```python
from build123d import *
from OCP.BRepAlgoAPI import BRepAlgoAPI_Cut
from OCP.TopTools import TopTools_ListOfShape

# Parameters (mm, degrees)
EXTRUDE_1_DEPTH        = 5
EXTRUDE_1_DEPTH_BACK   = 280.836309
SKETCH_1_R             = 12.5
HOLE_WIZARD_M101_D     = 8.5
HOLE_WIZARD_M101_DEPTH = 27.5
HOLE_WIZARD_M101_TIP   = 2.553657631
SKETCH_6_W             = 7
SKETCH_6_H             = 7
CUT_EXTRUDE_1_DEPTH    = 35
SKETCH_7_W             = 1.5
SKETCH_7_H             = 2.75
CUT_EXTRUDE_START      = -285.836309
SKETCH_6_2_W           = 7
SKETCH_6_2_H           = 7
CUT_EXTRUDE_2_DEPTH    = 31.8
HOLE_WIZARD_M102_D     = 8.5
HOLE_WIZARD_M102_DEPTH = 27.5
HOLE_WIZARD_M102_TIP   = 2.553657631


with BuildPart() as part:
    # Эскиз1 → Бобышка-Вытянуть1 (new, two sides: drawn at the far end of the back side and taken through both)
    with BuildSketch(Plane.XY.offset(-EXTRUDE_1_DEPTH_BACK)):
        Circle(SKETCH_1_R)
    extrude(amount=EXTRUDE_1_DEPTH + EXTRUDE_1_DEPTH_BACK)

    # Отверстие обработанное метчиком M101
    with Locations(Plane(origin=(0, 0, -280.836309448), x_dir=(-1, 0, 0), z_dir=(0, 0, -1))):
        with Locations((0, 0)):
            Hole(HOLE_WIZARD_M101_D / 2, depth=HOLE_WIZARD_M101_DEPTH)
            with Locations((0, 0, -(HOLE_WIZARD_M101_DEPTH + HOLE_WIZARD_M101_TIP / 2))):  # 118° drill point
                Cone(0, HOLE_WIZARD_M101_D / 2, HOLE_WIZARD_M101_TIP, mode=Mode.SUBTRACT)

    # Эскиз6 → Вырез-Вытянуть1 (cut)
    with BuildSketch(Plane(origin=(0, 0, -280.836309448), x_dir=(-1, 0, 0), z_dir=(0, 0, -1))):
        with Locations((0, 12.5)):
            Rectangle(SKETCH_6_W, SKETCH_6_H)
    extrude(amount=-CUT_EXTRUDE_1_DEPTH, mode=Mode.SUBTRACT)

    # Эскиз7 → Вырез-Повернуть1 (revolve, cut)
    with BuildSketch(Plane(origin=(0, 0, 0), x_dir=(0, 0, -1), z_dir=(1, 0, 0)), mode=Mode.PRIVATE) as cut_revolve_1_sk:
        with Locations((62.65, 13.125)):
            Rectangle(SKETCH_7_W, SKETCH_7_H)
        with Locations((27.55, 13.125)):
            Rectangle(SKETCH_7_W, SKETCH_7_H)
        with Locations((168.386309448, 13.125)):
            Rectangle(SKETCH_7_W, SKETCH_7_H)
    revolve(cut_revolve_1_sk.sketch.rotate(Axis((0, 0, 1000), (0, 0, -1)), 90), axis=Axis((0, 0, 1000), (0, 0, -1)), mode=Mode.SUBTRACT)


with BuildPart() as cut_extrude_2_tool:
    # Эскиз6<2> → Вырез-Вытянуть2 (new body)
    with BuildSketch(Plane(origin=(0, 0, -280.836309448), x_dir=(-1, 0, 0), z_dir=(0, 0, -1)).offset(CUT_EXTRUDE_START)):
        with Locations((0, 12.5)):
            Rectangle(SKETCH_6_2_W, SKETCH_6_2_H)
    extrude(amount=CUT_EXTRUDE_2_DEPTH)


with BuildPart() as part_1:
    add(part.part)

    # Вырез-Вытянуть2: cut by cut_extrude_2_tool, with a tolerance
    cut_extrude_2_stock = TopTools_ListOfShape()
    cut_extrude_2_stock.Append(part_1.part.wrapped)
    cut_extrude_2_tools = TopTools_ListOfShape()
    cut_extrude_2_tools.Append(cut_extrude_2_tool.part.wrapped)
    cut_extrude_2_cut = BRepAlgoAPI_Cut()
    cut_extrude_2_cut.SetArguments(cut_extrude_2_stock)
    cut_extrude_2_cut.SetTools(cut_extrude_2_tools)
    cut_extrude_2_cut.SetFuzzyValue(0.00001)
    cut_extrude_2_cut.Build()
    add(Compound.cast(cut_extrude_2_cut.Shape()).solids(), mode=Mode.REPLACE)

    # Отверстие обработанное метчиком M102
    with Locations(Plane.XY.offset(5)):
        with Locations((0, 0)):
            Hole(HOLE_WIZARD_M102_D / 2, depth=HOLE_WIZARD_M102_DEPTH)
            with Locations((0, 0, -(HOLE_WIZARD_M102_DEPTH + HOLE_WIZARD_M102_TIP / 2))):  # 118° drill point
                Cone(0, HOLE_WIZARD_M102_D / 2, HOLE_WIZARD_M102_TIP, mode=Mode.SUBTRACT)


solid = part_1.part
```
Source: CAD feature listing. Evaluate the final solid. Frame: model axes, mm. A direction names the side the tool comes from. Round coordinates to 2 decimals unless told otherwise and drop trailing zeros. Loops run counter-clockwise (first coordinate to the right, second up) from the corner with the lowest first, then second, coordinate; pieces in that order, holes last.
(1) Contact query for flat-ended pins moving along their axis: pin 1 Ø5.5 at (x, z) = (-1.5, -268.5) entering from +Y; pin 2 Ø10 at (x, z) = (8.5, -148) entering from -Y; pin 3 Ø4 at (y, z) = (6, -112.5) entering from -X. Output: stop coordinate, or through.
From the geometry:
pin 1: stops at y = 12
pin 2: stops at y = -12
pin 3: stops at x = -11.84
(2) Section query A-A (z = -259). Output: boundary loops of the cut face in (x, y), and give its area (3 significant figures).
From the geometry:
outline: (-3.5, 9) - (-3.5, 12) arc R12.5 ccw (long way) to (3.5, 12) - (3.5, 9) - close; hole circle Ø8.5 at (0, 0)
area: 411 mm2
(3) Pull-direction query (Z, two-part tool) for faces 1 (the cylindrical face through (-0.5, -12.49, -11.12)), 2 (the flat face through (-11, 5, -167.636)), 3 (the conical face through (-0.16, -0.72, -24.61)); classes: +Z half, -Z half, draft (parallel to the pull), parting line (faces both ways), or undercut.
From the geometry:
face 1: draft
face 2: undercut
face 3: +Z half
(4) Access query for faces 4 (the flat face through (-11, 5, -63.4)), 5 (the cylindrical face through (-2.285, 3.584, -8.943)), 6 (the cylindrical face through (2.285, 3.584, -266.894)), 7 (the flat face through (0, 9, -264)), 8 (the flat face through (0, 9, -11)). Directions: +Z, -Z, +X, -X, +Y, -Y. A direction counts if a zero-diameter tool reaches every point of the face in a straight line with its end or side. Return the directions, or none.
From the geometry:
face 4: none
face 5: +Z
face 6: -Z
face 7: -Z, +Y
face 8: +Z, +Y
(5) Section query C-C (z = -228). Output: boundary loops of the cut face in (x, y).
From the geometry:
outline: circle Ø25 at (0, 0)
(6) Section query B-B (y = -8). Output: boundary loops of the cut face in (x, z).
From the geometry:
outline: (-9.6, -280.84) - (9.6, -280.84) - (9.6, -169.14) - (8.61, -169.14) - (8.61, -167.64) - (9.6, -167.64) - (9.6, -63.4) - (8.61, -63.4) - (8.61, -61.9) - (9.6, -61.9) - (9.6, -28.3) - (8.61, -28.3) - (8.61, -26.8) - (9.6, -26.8) - (9.6, 5) - (-9.6, 5) - (-9.6, -26.8) - (-8.61, -26.8) - (-8.61, -28.3) - (-9.6, -28.3) - (-9.6, -61.9) - (-8.61, -61.9) - (-8.61, -63.4) - (-9.6, -63.4) - (-9.6, -167.64) - (-8.61, -167.64) - (-8.61, -169.14) - (-9.6, -169.14) - close
(7) Material intervals for probe 1 along X at (y, z) = (0, -265.75); probe 2 along Y at (x, z) = (0, -8.5); probe 3 along Y at (x, z) = (-3, -18.5), sorted ascending.
From the geometry:
probe 1: x = -12.5 to -4.25, 4.25 to 12.5
probe 2: y = -12.5 to -4.25, 4.25 to 9
probe 3: y = -12.13 to -3.01, 3.01 to 9
